Here's how the part is built. I have some questions about the finished solid (model axes, mm). A direction names the side the tool comes from. Round coordinates to 2 decimals unless told otherwise and drop trailing zeros. Order: outer loops, then holes, each group sorted by start corner. A loop starts at its lowest first (then second) coordinate and runs counter-clockwise, first axis right, second up. Notation, with made-up numbers: (-38, 43) - (2, 43) arc R19 ccw to (2, 70) - close; hole circle Ø8 at (18, -29.5). An arc over 180 degrees is marked (long way). One line per item, written item: value.
from build123d import *

# Parameters (mm, degrees)
SKETCH4_R            = 1.5
SKETCH4_W            = 25.4
SKETCH4_H            = 4.6
SKETCH4_W_2          = 6.1
SKETCH4_W_3          = 4
SKETCH4_H_2          = 4
BOSS_EXTRUDE1_DEPTH  = 1.5
SKETCH4_4_W          = 6.1
SKETCH4_4_H          = 4.6
BOSS_EXTRUDE3_DEPTH  = 6.75
BOSS_EXTRUDE4_START  = -6.75
SKETCH4_5_R          = 3.25
BOSS_EXTRUDE4_DEPTH  = 1.5
BOSS_EXTRUDE5_START  = -6.75
SKETCH4_7_R          = 4.25
SKETCH4_7_R_2        = 3.25
BOSS_EXTRUDE5_DEPTH  = 1
SKETCH5_R            = 5.25
SKETCH5_R_2          = 1.5
BOSS_EXTRUDE6_DEPTH  = 1
BOSS_EXTRUDE7_START  = 31.5
SKETCH4_9_R          = 1.25
SKETCH4_9_R_2        = 5
SKETCH4_9_R_3        = 1.5
SKETCH4_9_W          = 6.1
SKETCH4_9_H          = 4.6
SKETCH4_9_W_2        = 25.4
SKETCH4_9_W_3        = 4
SKETCH4_9_H_2        = 4
BOSS_EXTRUDE7_DEPTH  = 1.5
BOSS_EXTRUDE8_START  = 1.5
SKETCH4_11_W         = 4
SKETCH4_11_H         = 4
BOSS_EXTRUDE8_DEPTH  = 30
BOSS_EXTRUDE9_START  = -8.25
BOSS_EXTRUDE9_DEPTH  = 41.25
FILLET1_R            = 1
BOSS_EXTRUDE10_REACH = 127.173
FILLET3_R            = 1


with BuildPart() as part:
    # Sketch4 → Boss-Extrude1 (new body)
    with BuildSketch(Plane(origin=(0, 0, 0), x_dir=(0, 0, -1), z_dir=(1, 0, 0))):
        with BuildLine():
            Line((12.7, 113.1), (12.7, 75.1))
            Line((12.7, 75.1), (18.8, 75.1))
            Line((18.8, 75.1), (18.8, 85.6))
            Line((18.8, 85.6), (18.8, 89.6))
            Line((18.8, 89.6), (18.8, 102.6))
            Line((18.8, 102.6), (18.8, 106.6))
            Line((18.8, 106.6), (18.8, 115.6))
            Line((18.8, 115.6), (15, 115.6))
            ThreePointArc((15, 115.6), (13.621502583, 115.185604198), (12.7, 114.079795897))
            Line((12.7, 114.079795897), (12.7, 113.1))
        make_face()
        with Locations((15, 79.1)):
            Circle(SKETCH4_R, mode=Mode.SUBTRACT)
        with Locations((15, 96.1)):
            Circle(SKETCH4_R, mode=Mode.SUBTRACT)
        with Locations((15, 113.1)):
            Circle(SKETCH4_R, mode=Mode.SUBTRACT)
        with Locations((0, 72.8)):
            Rectangle(SKETCH4_W, SKETCH4_H)
        with Locations((-8.5, 72.8)):
            Circle(SKETCH4_R, mode=Mode.SUBTRACT)
        with Locations((8.5, 72.8)):
            Circle(SKETCH4_R, mode=Mode.SUBTRACT)
        with BuildLine():
            Line((-18.8, 75.1), (-12.7, 75.1))
            Line((-12.7, 75.1), (-12.7, 113.1))
            Line((-12.7, 113.1), (-12.7, 114.079795897))
            ThreePointArc((-12.7, 114.079795897), (-13.621502583, 115.185604198), (-15, 115.6))
            Line((-15, 115.6), (-18.8, 115.6))
            Line((-18.8, 115.6), (-18.8, 106.6))
            Line((-18.8, 106.6), (-18.8, 102.6))
            Line((-18.8, 102.6), (-18.8, 89.6))
            Line((-18.8, 89.6), (-18.8, 85.6))
            Line((-18.8, 85.6), (-18.8, 75.1))
        make_face()
        with Locations((-15, 79.1)):
            Circle(SKETCH4_R, mode=Mode.SUBTRACT)
        with Locations((-15, 96.1)):
            Circle(SKETCH4_R, mode=Mode.SUBTRACT)
        with Locations((-15, 113.1)):
            Circle(SKETCH4_R, mode=Mode.SUBTRACT)
        with Locations((15.75, 72.8)):
            Rectangle(SKETCH4_W_2, SKETCH4_H)
        with Locations((-15.75, 72.8)):
            Rectangle(SKETCH4_W_2, SKETCH4_H)
        with Locations((-20.8, 87.6)):
            Rectangle(SKETCH4_W_3, SKETCH4_H_2)
        with Locations((-20.8, 104.6)):
            Rectangle(SKETCH4_W_3, SKETCH4_H_2)
        with Locations((20.8, 104.6)):
            Rectangle(SKETCH4_W_3, SKETCH4_H_2)
        with Locations((20.8, 87.6)):
            Rectangle(SKETCH4_W_3, SKETCH4_H_2)
    extrude(amount=BOSS_EXTRUDE1_DEPTH)

    # Sketch4_4 → Boss-Extrude3 (add)
    with BuildSketch(Plane(origin=(0, 0, 0), x_dir=(0, 0, -1), z_dir=(1, 0, 0))):
        with Locations((15.75, 72.8)):
            Rectangle(SKETCH4_4_W, SKETCH4_4_H)
        with Locations((-15.75, 72.8)):
            Rectangle(SKETCH4_4_W, SKETCH4_4_H)
    extrude(amount=-BOSS_EXTRUDE3_DEPTH)

    # Sketch4_5 → Boss-Extrude4 (add)
    with BuildSketch(Plane(origin=(0, 0, 0), x_dir=(0, 0, -1), z_dir=(1, 0, 0)).offset(BOSS_EXTRUDE4_START)):
        with BuildLine():
            Line((-12.7, 70.5), (-12.7, 75.1))
            Line((-12.7, 75.1), (-18.8, 75.1))
            Line((-18.8, 75.1), (-18.8, 70))
            Line((-18.8, 70), (-10.933485156, -1.207850299))
            ThreePointArc((-10.933485156, -1.207850299), (0, -11), (10.933485156, -1.207850299))
            Line((10.933485156, -1.207850299), (18.8, 70))
            Line((18.8, 70), (18.8, 75.1))
            Line((18.8, 75.1), (12.7, 75.1))
            Line((12.7, 75.1), (12.7, 70.5))
            Line((12.7, 70.5), (-12.7, 70.5))
        make_face()
        Circle(SKETCH4_5_R, mode=Mode.SUBTRACT)
    extrude(amount=-BOSS_EXTRUDE4_DEPTH)

    # Sketch4_7 → Boss-Extrude5 (add)
    with BuildSketch(Plane(origin=(0, 0, 0), x_dir=(0, 0, -1), z_dir=(1, 0, 0)).offset(BOSS_EXTRUDE5_START)):
        Circle(SKETCH4_7_R)
        Circle(SKETCH4_7_R_2, mode=Mode.SUBTRACT)
    extrude(amount=BOSS_EXTRUDE5_DEPTH)

    # Sketch5 → Boss-Extrude6 (add)
    with BuildSketch(Plane.ZY.offset(8.25)):
        with Locations(Location((0, 0, 0), (0, 0, 180))):
            Circle(SKETCH5_R)
        Circle(SKETCH5_R_2, mode=Mode.SUBTRACT)
    extrude(amount=BOSS_EXTRUDE6_DEPTH)



with BuildPart() as body_2:
    # Sketch4_9 → Boss-Extrude7 (new body)
    with BuildSketch(Plane(origin=(0, 0, 0), x_dir=(0, 0, -1), z_dir=(1, 0, 0)).offset(BOSS_EXTRUDE7_START)):
        with BuildLine():
            Line((12.7, 70.5), (-12.7, 70.5))
            Line((-12.7, 70.5), (-18.8, 70.5))
            Line((-18.8, 70.5), (-18.8, 70))
            Line((-18.8, 70), (-18.467246252, 66.987906392))
            Line((-18.467246252, 66.987906392), (-18.028027961, 63.012093608))
            Line((-18.028027961, 63.012093608), (-14.600705998, 31.987906392))
            Line((-14.600705998, 31.987906392), (-14.161487708, 28.012093608))
            Line((-14.161487708, 28.012093608), (-10.933485156, -1.207850299))
            ThreePointArc((-10.933485156, -1.207850299), (0, -11), (10.933485156, -1.207850299))
            Line((10.933485156, -1.207850299), (14.161487708, 28.012093608))
            Line((14.161487708, 28.012093608), (14.600705998, 31.987906392))
            Line((14.600705998, 31.987906392), (18.028027961, 63.012093608))
            Line((18.028027961, 63.012093608), (18.467246252, 66.987906392))
            Line((18.467246252, 66.987906392), (18.8, 70))
            Line((18.8, 70), (18.8, 70.5))
            Line((18.8, 70.5), (12.7, 70.5))
        make_face()
        with Locations((-8, 0)):
            Circle(SKETCH4_9_R, mode=Mode.SUBTRACT)
        with Locations((-5.656854249, -5.656854249)):
            Circle(SKETCH4_9_R, mode=Mode.SUBTRACT)
        Circle(SKETCH4_9_R_2, mode=Mode.SUBTRACT)
        with Locations((-5.656854249, 5.656854249)):
            Circle(SKETCH4_9_R, mode=Mode.SUBTRACT)
        with Locations((0, 8)):
            Circle(SKETCH4_9_R, mode=Mode.SUBTRACT)
        with Locations((0, -8)):
            Circle(SKETCH4_9_R, mode=Mode.SUBTRACT)
        with Locations((5.656854249, -5.656854249)):
            Circle(SKETCH4_9_R, mode=Mode.SUBTRACT)
        with Locations((8, 0)):
            Circle(SKETCH4_9_R, mode=Mode.SUBTRACT)
        with Locations((5.656854249, 5.656854249)):
            Circle(SKETCH4_9_R, mode=Mode.SUBTRACT)
        with BuildLine():
            Line((-18.8, 75.1), (-12.7, 75.1))
            Line((-12.7, 75.1), (-12.7, 113.1))
            Line((-12.7, 113.1), (-12.7, 114.079795897))
            ThreePointArc((-12.7, 114.079795897), (-13.621502583, 115.185604198), (-15, 115.6))
            Line((-15, 115.6), (-18.8, 115.6))
            Line((-18.8, 115.6), (-18.8, 106.6))
            Line((-18.8, 106.6), (-18.8, 102.6))
            Line((-18.8, 102.6), (-18.8, 89.6))
            Line((-18.8, 89.6), (-18.8, 85.6))
            Line((-18.8, 85.6), (-18.8, 75.1))
        make_face()
        with Locations((-15, 79.1)):
            Circle(SKETCH4_9_R_3, mode=Mode.SUBTRACT)
        with Locations((-15, 96.1)):
            Circle(SKETCH4_9_R_3, mode=Mode.SUBTRACT)
        with Locations((-15, 113.1)):
            Circle(SKETCH4_9_R_3, mode=Mode.SUBTRACT)
        with Locations((-15.75, 72.8)):
            Rectangle(SKETCH4_9_W, SKETCH4_9_H)
        with Locations((15.75, 72.8)):
            Rectangle(SKETCH4_9_W, SKETCH4_9_H)
        with Locations((0, 72.8)):
            Rectangle(SKETCH4_9_W_2, SKETCH4_9_H)
        with Locations((-8.5, 72.8)):
            Circle(SKETCH4_9_R_3, mode=Mode.SUBTRACT)
        with Locations((8.5, 72.8)):
            Circle(SKETCH4_9_R_3, mode=Mode.SUBTRACT)
        with BuildLine():
            Line((12.7, 113.1), (12.7, 75.1))
            Line((12.7, 75.1), (18.8, 75.1))
            Line((18.8, 75.1), (18.8, 85.6))
            Line((18.8, 85.6), (18.8, 89.6))
            Line((18.8, 89.6), (18.8, 102.6))
            Line((18.8, 102.6), (18.8, 106.6))
            Line((18.8, 106.6), (18.8, 115.6))
            Line((18.8, 115.6), (15, 115.6))
            ThreePointArc((15, 115.6), (13.621502583, 115.185604198), (12.7, 114.079795897))
            Line((12.7, 114.079795897), (12.7, 113.1))
        make_face()
        with Locations((15, 79.1)):
            Circle(SKETCH4_9_R_3, mode=Mode.SUBTRACT)
        with Locations((15, 96.1)):
            Circle(SKETCH4_9_R_3, mode=Mode.SUBTRACT)
        with Locations((15, 113.1)):
            Circle(SKETCH4_9_R_3, mode=Mode.SUBTRACT)
        with Locations((-20.8, 104.6)):
            Rectangle(SKETCH4_9_W_3, SKETCH4_9_H_2)
        with Locations((-20.8, 87.6)):
            Rectangle(SKETCH4_9_W_3, SKETCH4_9_H_2)
        with Locations((20.8, 104.6)):
            Rectangle(SKETCH4_9_W_3, SKETCH4_9_H_2)
        with Locations((20.8, 87.6)):
            Rectangle(SKETCH4_9_W_3, SKETCH4_9_H_2)
    extrude(amount=BOSS_EXTRUDE7_DEPTH)


with BuildPart() as part_1:
    add(part.part)

    add(body_2.part)  # Boss-Extrude8 merges body 2
    # Sketch4_11 → Boss-Extrude8 (add)
    with BuildSketch(Plane(origin=(0, 0, 0), x_dir=(0, 0, -1), z_dir=(1, 0, 0)).offset(BOSS_EXTRUDE8_START)):
        with Locations((-20.8, 87.6)):
            Rectangle(SKETCH4_11_W, SKETCH4_11_H)
        with Locations((-20.8, 104.6)):
            Rectangle(SKETCH4_11_W, SKETCH4_11_H)
        with Locations((20.8, 104.6)):
            Rectangle(SKETCH4_11_W, SKETCH4_11_H)
        with Locations((20.8, 87.6)):
            Rectangle(SKETCH4_11_W, SKETCH4_11_H)
    extrude(amount=BOSS_EXTRUDE8_DEPTH)

    # Sketch4_12 → Boss-Extrude9 (add)
    with BuildSketch(Plane(origin=(0, 0, 0), x_dir=(0, 0, -1), z_dir=(1, 0, 0)).offset(BOSS_EXTRUDE9_START)):
        Polygon((22.443059036, 66.548688101), (18.467246252, 66.987906392), (18.028027961, 63.012093608), (22.003840745, 62.572875317), align=None)
        Polygon((18.576518782, 31.548688101), (14.600705998, 31.987906392), (14.161487708, 28.012093608), (18.137300492, 27.572875317), align=None)
    extrude(amount=BOSS_EXTRUDE9_DEPTH)

    # Fillet1
    fillet1_edges = [part_1.edges().sort_by_distance(p)[0] for p in [
        (32.25, 115.6, 18.8),
        (32.25, 115.6, -18.8),
        (0.75, 115.6, -18.8),
        (0.75, 115.6, 18.8),
        (16.5, 89.6, 22.8),
        (16.5, 85.6, 22.8),
        (16.5, 106.6, 22.8),
        (16.5, 102.6, 22.8),
        (16.5, 102.6, -22.8),
        (16.5, 106.6, -22.8),
        (16.5, 85.6, -22.8),
        (16.5, 89.6, -22.8),
    ]]
    fillet(fillet1_edges, radius=FILLET1_R)

    # Boss-Extrude10: up to this face of the body (flat: up to its plane)
    boss_extrude10_end = Plane(part_1.part.faces().sort_by_distance((-8.25, 37.164780502, -0.254514777))[0])
    # Sketch6 → Boss-Extrude10 (add, up to the picked face)
    with BuildSketch(Plane(origin=(33, 0, 0), x_dir=(0, 0, -1), z_dir=(1, 0, 0)), mode=Mode.PRIVATE) as boss_extrude10_sk1:
        Polygon((16.094757835, 45.512093608), (16.533976125, 49.487906392), (20.509788909, 49.048688101), (20.070570619, 45.072875318), align=None)
    boss_extrude10_tool1 = split(extrude(boss_extrude10_sk1.sketch, amount=-BOSS_EXTRUDE10_REACH, mode=Mode.PRIVATE), bisect_by=boss_extrude10_end, keep=Keep.BOTH, mode=Mode.PRIVATE)
    add(boss_extrude10_tool1.solids().sort_by(Axis((33, 47.280391, -18.302273), (-1, 0, 0)))[0])

    # Fillet3
    fillet3_edges = [part_1.edges().sort_by_distance(p)[0] for p in [
        (12.375, 66.548688101, -22.443059036),
        (12.375, 62.572875317, -22.003840745),
        (12.375, 31.548688101, -18.576518782),
        (12.375, 27.572875317, -18.137300492),
        (12.375, 45.072875318, -20.070570619),
        (12.375, 49.048688101, -20.509788909),
    ]]
    fillet(fillet3_edges, radius=FILLET3_R)


solid = part_1.part
Q1. If we section it at A-A, the plane x = -2.5: Please give me the cut outline in (y, z).
Results list:
outline: (27.68, -17.14) arc R1 ccw to (28.57, -18.25) - (30.55, -18.47) arc R1 ccw to (31.66, -17.58) - (31.99, -14.6) - (28.01, -14.16) - close; (45.18, -19.08) arc R1 ccw to (46.07, -20.18) - (48.05, -20.4) arc R1 ccw to (49.16, -19.52) - (49.49, -16.53) - (45.51, -16.09) - close; (62.68, -21.01) arc R1 ccw to (63.57, -22.11) - (65.55, -22.33) arc R1 ccw to (66.66, -21.45) - (66.99, -18.47) - (63.01, -18.03) - close; (70.5, -18.8) - (75.1, -18.8) - (75.1, -12.7) - (70.5, -12.7) - close; (70.5, 12.7) - (75.1, 12.7) - (75.1, 18.8) - (70.5, 18.8) - close
Q2. Which directions (+Z, -Z, +X, -X, +Y, -Y) give clear straight access to the entire face, cutting with the end or side of a thin tool? Please do faces 4 (the cylindrical face through (-8.7, -1.6, -5)), 5 (the cylindrical face through (0.74, 77.636, 15.325)), 6 (the flat face through (16, 88, 18.8)), 7 (the flat face through (-4, 73, -12.7)), 8 (the cylindrical face through (32.24, 4.55, 5.08)).
Results list:
face 4: -X
face 5: +X, -X
face 6: +Y, -Y
face 7: -X, +Y
face 8: +X
Q3. If we section it at C-C, the plane y = 43: Please give me the cut outline in (x, z).
Results list:
outline: (-8.25, -15.82) - (-6.75, -15.82) - (-6.75, 15.82) - (-8.25, 15.82) - close; (31.5, -15.82) - (33, -15.82) - (33, 15.82) - (31.5, 15.82) - close
Q4. If I drill on line 1 along Z through (x, y) = (32.55, 113.1); line 2 along X through (y, z) = (104, 13); line 3 along X through (y, z) = (16, -8.5), over which ranges is the centre line in solid material (lowest first)?
Results list:
line 1: -18.8 to -16.5, -13.5 to -12.7, 12.7 to 13.5, 16.5 to 18.8
line 2: 0 to 1.5, 31.5 to 33
line 3: -8.25 to -6.75, 31.5 to 33
Q5. We'd pull the mould along Y, two halves only. Please class faces 1 (the flat face through (16, 102.6, -20)), 2 (the flat face through (16, 105, 18.8)), 3 (the flat face through (16, 106.6, 20)): released by +Y, released by -Y, zero draft, split by the parting line, or undercut.
Results list:
face 1: undercut
face 2: zero draft
face 3: released by +Y
Q6. Will these pins go through, and if not, where does the flat tip stop? pin 1 (12 mm diameter, centred on x = 4, y = 74, fed in from +Z); pin 2 (12 mm diameter, centred on x = -4, y = 64.5, fed in from -Z); pin 3 (10 mm diameter, centred on x = 19, z = -16.5, fed in from +Y).
Results list:
pin 1: z = 18.8
pin 2: z = -22.34
pin 3: y = 106.6
Q7. If we section it at B-B, the plane z = 20: Please give me the cut outline in (x, y).
Results list:
outline: (0, 85.6) - (33, 85.6) - (33, 89.6) - (0, 89.6) - close; (0, 102.6) - (33, 102.6) - (33, 106.6) - (0, 106.6) - close
Q8. If we section it at D-D, the plane z = 0: Give the number of separate pieces and of enclosed holes in the cut face, then the cut area to 3 significant figures.
Results list:
separate pieces: 7
enclosed holes: 0
area: 236 mm²
